```python
from build123d import *

# Parameters (mm, degrees)
SKETCH_1_R      = 2
EXTRUDE_1_DEPTH = 3


with BuildPart() as part:
    # 草图1 → 凸台-拉伸1 (new body)
    with BuildSketch(Plane(origin=(0, 0, 0), x_dir=(1, 0, 0), z_dir=(0, 1, 0))):
        Polygon((0, 3.914434825), (-3.39, 1.957217413), (-3.39, -1.957217413), (0, -3.914434825), (3.39, -1.957217413), (3.39, 1.957217413), align=None)
        with Locations(Location((0, 0, 0), (0, 0, 270))):
            Circle(SKETCH_1_R, mode=Mode.SUBTRACT)
    extrude(amount=EXTRUDE_1_DEPTH)

    # 草图12 → 切除-旋转1 (revolve, cut)
    with BuildSketch(Plane(origin=(0, 0, 0), x_dir=(-0.8660254037844386, 0, -0.5000000000000003), z_dir=(0.5000000000000002, 0, -0.8660254037844385))):
        Polygon((-3.414434825, 3), (-3.914434825, 2.5), (-3.914434825, 3), align=None)
    cut_revolve_1 = revolve(axis=Axis((0, 3, 0), (0, 1, 0)), mode=Mode.SUBTRACT)

    # 镜向1: 切除-旋转1 across plane
    add(cut_revolve_1.mirror(Plane.ZX.offset(1.5)), mode=Mode.SUBTRACT)


solid = part.part
```
Can you work these out from the model? Positions are in its coordinate system, mm. Give positions to 0.01 mm unless a question says otherwise; leave off trailing zeros. Loops run counter-clockwise (first coordinate to the right, second up) from the corner with the lowest first, then second, coordinate; pieces in that order, holes last. Notation, with made-up numbers: M -26.5,37 L -0.5,37 A32 cw -0.5,66 Z; hole C -10,-37 d8. An arc over 180 degrees is marked long. Use one line per item in the form item = value. Start each with the question number.
(1) I want a section at A-A, the plane z = 0. Write out the boundary of the cut face in (x, y).
(2) I want a section at B-B, the plane y = 1.45. Write out the boundary of the cut face in (x, z).
(3) I'm going to push a flat-ended pin straight in: P1, Ø2.5, axis at x = 0, z = 0, coming from the +Y side. Where does the tip first touch, or does it pass through?
(4) I want a section at D-D, the plane y = 2.65. Write out the boundary of the cut face in (x, z).
(5) I want a section at C-C, the plane x = 1.5. Write out the boundary of the cut face in (y, z).
(6) Please list where these lines run through material, in increasing order: line 1 (X direction, y = 1, z = 0); line 2 (Z direction, x = -0.25, y = 2.25); line 3 (Z direction, x = 1.25, y = 1.55).
(7) Thinking about a two-plate mould opening in Z: for faces 1 (the cylindrical face through (-2, 1, 0)), 2 (the flat face through (3.39, 1, 0)), 3 (the conical face through (3.09, 2.86, -1.76)), 4 (the conical face through (-3.09, 0.14, 1.76)), which applies, released by +Z, released by -Z, zero draft, split by the parting line, or undercut?
Worked out:
q1.outline = M -3.39,0 L -2,0 L -2,3 L -3.39,3 Z; M 2,0 L 3.39,0 L 3.39,3 L 2,3 Z
q2.outline = M -3.39,-1.96 L 0,-3.91 L 3.39,-1.96 L 3.39,1.96 L 0,3.91 L -3.39,1.96 Z; hole C 0,0 d4
q3.P1 = through
q4.outline = M -3.39,-1.64 A3.76 ccw -3.11,-2.12 L -0.28,-3.75 A3.76 ccw 0.28,-3.75 L 3.11,-2.12 A3.76 ccw 3.39,-1.64 L 3.39,1.64 A3.76 ccw 3.11,2.12 L 0.28,3.75 A3.76 ccw -0.28,3.75 L -3.11,2.12 A3.76 ccw -3.39,1.64 Z; hole C 0,0 d4
q5.outline = M 0,-3.05 L 3,-3.05 L 3,-1.32 L 0,-1.32 Z; M 0,1.32 L 3,1.32 L 3,3.05 L 0,3.05 Z
q6.line_1 = -3.39 to -2, 2 to 3.39
q6.line_2 = -3.77 to -1.98, 1.98 to 3.77
q6.line_3 = -3.19 to -1.56, 1.56 to 3.19
q7.face_1 = undercut
q7.face_2 = zero draft
q7.face_3 = released by -Z
q7.face_4 = released by +Z
